Part model, mm, in its own coordinate system. A direction names the side the tool comes from. Give positions to 0.01 mm unless a question says otherwise; leave off trailing zeros. Write each loop counter-clockwise with the first axis right and the second up, starting at its lowest first coordinate (ties: lowest second). Pieces come first, ordered by that corner, then holes. Notation, with made-up numbers: M 64,28 L 69,28 A28 cw 69,63 Z; hole C -31,79 d2. An arc over 180 degrees is marked long. Use CSV: the item, a comma, the result in double quotes. Start each with the question number.
Item 1: Drill centre lines: line 1 (Z direction, x = -24, y = -1.5); line 2 (X direction, y = 1.5, z = -5); line 3 (X direction, y = 2.5, z = 6). Where is each one in solid material? Low to high. Write a range as [from, to].
Item 2: Which spindle directions (+Z, -Z, +X, -X, +Y, -Y) get a long thin tool onto all of the face, cutting with end or side? Do faces 1 (the cylindrical face through (10.165, -1.014, -9.699)), 2 (the flat face through (-10, 3, 9)), 3 (the cylindrical face through (-29.649, -1.014, -9.715)), 4 (the flat face through (-18, 10, 0)), 5 (the flat face through (-12, 9.5, 0)). Say none if no direction does.
Item 3: Mould opens along Z. For faces 6 (the cylindrical face through (13.5, 0.99, 4.93)), 7 (the cylindrical face through (10.165, 4.014, -9.699)), 8 (the flat face through (10.45, 4, 0)), 9 (the cylindrical face through (-37.215, 1.014, 9.699)) say: released by +Z, released by -Z, zero draft, split by the parting line, or undercut.
Item 4: Cut at B-B (y = -1). List the corners of the cut face in (x, z).
Item 5: Cut at A-A (x = -35). List the corners of the cut face in (y, z), then the cut area to 3 significant figures.
Item 6: Pin check, flat tips, straight feed: pin 1 (0.6 mm diameter, centred on x = -37.5, y = 1.5, fed in from -Z); pin 2 (1.7 mm diameter, centred on y = 3, z = 3.5, fed in from -X); pin 3 (4 mm diameter, centred on y = 6, z = -5.5, fed in from -X); pin 4 (3 mm diameter, centred on x = -35, z = -5, fed in from +Y). Stop position of each tip, or through.
from build123d import *

# Parameters (mm, degrees)
ESQUISSE1_W              = 38.4
ESQUISSE1_H              = 18
BOSS_EXTRU_1_DEPTH       = 2
ESQUISSE2_W              = 40.4
ESQUISSE2_H              = 20
ESQUISSE2_W_2            = 38.4
ESQUISSE2_H_2            = 18
BOSS_EXTRU_2_DEPTH       = 2
EXTRU_MINCE1_DEPTH       = 10
EXTRU_MINCE1_DEPTH_BACK  = 10
BOSS_EXTRU_3_DEPTH       = 1
ESQUISSE6_R              = 2.65
ENL_V_MAT_EXTRU_1_DEPTH  = 41.929818
BOSS_EXTRU_7_START       = -9
BOSS_EXTRU_7_DEPTH       = 18
BOSS_EXTRU_7_2_OUTLINE_W = 18
BOSS_EXTRU_7_2_OUTLINE_H = 0.5
BOSS_EXTRU_7_2_DEPTH     = 6.350393
BOSS_EXTRU_7_START_2     = 2.65
BOSS_EXTRU_7_3_OUTLINE_W = 18
BOSS_EXTRU_7_3_OUTLINE_H = 0.5
BOSS_EXTRU_7_3_DEPTH     = 6.35
BOSS_EXTRU_7_START_3     = 9.5
BOSS_EXTRU_7_4_DEPTH     = 0.5
BOSS_EXTRU_7_5_DEPTH     = 0.5
CONG_1_R                 = 1
ENL_V_MAT_EXTRU_2_DEPTH  = 44.453999


with BuildPart() as part:
    # Esquisse1 → Boss.-Extru.1 (new body)
    with BuildSketch(Plane(origin=(0, 0, 0), x_dir=(1, 0, 0), z_dir=(0, 1, 0))):
        with BuildLine():
            Line((-37.5, 10), (18, 10))
            Line((18, 10), (18, 6))
            Line((18, 6), (17.232051, 6))
            ThreePointArc((17.232051, 6), (13.5, 5), (17.232051, 4))
            Line((17.232051, 4), (18, 4))
            Line((18, 4), (18, -4))
            Line((18, -4), (17.232051, -4))
            ThreePointArc((17.232051, -4), (13.5, -5), (17.232051, -6))
            Line((17.232051, -6), (18, -6))
            Line((18, -6), (18, -10))
            Line((18, -10), (-37.5, -10))
            Line((-37.5, -10), (-37.5, -6))
            Line((-37.5, -6), (-36.732051, -6))
            ThreePointArc((-36.732051, -6), (-33, -5), (-36.732051, -4))
            Line((-36.732051, -4), (-37.5, -4))
            Line((-37.5, -4), (-37.5, 4))
            Line((-37.5, 4), (-36.732051, 4))
            ThreePointArc((-36.732051, 4), (-33, 5), (-36.732051, 6))
            Line((-36.732051, 6), (-37.5, 6))
            Line((-37.5, 6), (-37.5, 10))
        make_face()
        with Locations((-9.75, 0)):
            Rectangle(ESQUISSE1_W, ESQUISSE1_H, mode=Mode.SUBTRACT)
    extrude(amount=BOSS_EXTRU_1_DEPTH)

    # Esquisse2 → Boss.-Extru.2 (add)
    with BuildSketch(Plane.XZ):
        with Locations((-9.75, 0)):
            Rectangle(ESQUISSE2_W, ESQUISSE2_H)
        with Locations((-9.75, 0)):
            Rectangle(ESQUISSE2_W_2, ESQUISSE2_H_2, mode=Mode.SUBTRACT)
    extrude(amount=BOSS_EXTRU_2_DEPTH)

    # Esquisse3 → Extru.-Mince1 (add, two sides: drawn at the far end of the back side and taken through both)
    with BuildSketch(Plane.XY.offset(-EXTRU_MINCE1_DEPTH_BACK)):
        Polygon((-29.95, 2), (-29.95, 4.786585), (-17, 9.5), (7.45, 9.5), (10.45, 6.5), (10.45, 2), (9.45, 2), (9.45, 6.085786), (7.035786, 8.5), (-16.823673, 8.5), (-28.95, 4.086378), (-28.95, 2), align=None)
    extrude(amount=EXTRU_MINCE1_DEPTH + EXTRU_MINCE1_DEPTH_BACK)

    # Esquisse4 → Boss.-Extru.3 (add)
    with BuildSketch(Plane.XY.offset(10)):
        Polygon((10.45, 6.5), (10.45, 2), (-29.95, 2), (-29.95, 4.786585), (-17, 9.5), (7.45, 9.5), align=None)
    boss_extru_3 = extrude(amount=-BOSS_EXTRU_3_DEPTH)

    # Symétrie1: Boss.-Extru.3 across plane
    add(boss_extru_3.mirror(Plane.XY))

    # Esquisse5 → Révolution1 (revolve)
    with BuildSketch(Plane.XY, mode=Mode.PRIVATE) as r_volution1_sk:
        Polygon((-6.25, 9.5), (-4.75, 11), (0, 11), (0, 10), (-4.335786, 10), (-5.542893, 8.792893), align=None)
    revolve(r_volution1_sk.sketch.rotate(Axis((0, 11, 0), (0, -1, 0)), 270), axis=Axis((0, 11, 0), (0, -1, 0)))

    # Esquisse6 → Enlèv. mat.-Extru.1 (cut, through all)
    with BuildSketch(Plane(origin=(0, 11, 0), x_dir=(1, 0, 0), z_dir=(0, 1, 0))):
        Circle(ESQUISSE6_R)
    extrude(amount=-ENL_V_MAT_EXTRU_1_DEPTH, mode=Mode.SUBTRACT)

    # Boss.-Extru.7: read off the stored shape, not the designer's step
    # Boss.-Extru.7 outline → Boss.-Extru.7 (add)
    with BuildSketch(Plane.XY.offset(BOSS_EXTRU_7_START)):
        Polygon((-12.5, 10), (-26.95, 10), (-26.95, 5.878496), (-17, 9.5), (-12.5, 9.5), align=None)
    extrude(amount=BOSS_EXTRU_7_DEPTH)

    # Boss.-Extru.7 2 outline → Boss.-Extru.7 2 (add)
    with BuildSketch(Plane.XY.offset(BOSS_EXTRU_7_START)):
        with Locations((-2.5, 9.75)):
            Rectangle(BOSS_EXTRU_7_2_OUTLINE_W, BOSS_EXTRU_7_2_OUTLINE_H)
    extrude(amount=BOSS_EXTRU_7_2_DEPTH)

    # Boss.-Extru.7 3 outline → Boss.-Extru.7 3 (add)
    with BuildSketch(Plane.XY.offset(BOSS_EXTRU_7_START_2)):
        with Locations((-2.5, 9.75)):
            Rectangle(BOSS_EXTRU_7_3_OUTLINE_W, BOSS_EXTRU_7_3_OUTLINE_H)
    extrude(amount=BOSS_EXTRU_7_3_DEPTH)

    # Boss.-Extru.7 4 outline → Boss.-Extru.7 4 (cut)
    with BuildSketch(Plane(origin=(0, 0, 0), x_dir=(1, 0, 0), z_dir=(0, 1, 0)).offset(BOSS_EXTRU_7_START_3)):
        with BuildLine():
            Line((-0.04562, 2.649607), (0.04562, 2.649607))
            ThreePointArc((0.04562, 2.649607), (0, 2.65), (-0.04562, 2.649607))
        make_face()
    extrude(amount=BOSS_EXTRU_7_4_DEPTH, mode=Mode.SUBTRACT)

    # Boss.-Extru.7 5 outline → Boss.-Extru.7 5 (add)
    with BuildSketch(Plane(origin=(0, 0, 0), x_dir=(1, 0, 0), z_dir=(0, 1, 0)).offset(BOSS_EXTRU_7_START_3)):
        with BuildLine():
            ThreePointArc((0.04562, 2.649607), (2.649902, -0.022811), (0, -2.65))
            Line((0, -2.65), (6.5, -2.65))
            Line((6.5, -2.65), (6.5, 2.649607))
            Line((6.5, 2.649607), (0.04562, 2.649607))
        make_face()
        with BuildLine():
            Line((-11.5, -2.65), (0, -2.65))
            ThreePointArc((0, -2.65), (-2.649902, -0.022811), (-0.04562, 2.649607))
            Line((-0.04562, 2.649607), (-11.5, 2.649607))
            Line((-11.5, 2.649607), (-11.5, -2.65))
        make_face()
    extrude(amount=BOSS_EXTRU_7_5_DEPTH)

    # Congé1
    cong_1_edges = [part.edges().sort_by_distance(p)[0] for p in [
        (-29.95, 4.786585, 0),
        (-23.475, 7.143293, -10),
        (-23.475, 7.143293, 10),
        (-4.775, 9.5, 10),
        (-4.775, 9.5, -10),
        (7.45, 9.5, 0),
        (10.45, 6.5, 0),
        (8.95, 8, 10),
        (8.95, 8, -10),
        (10.45, 4.25, 10),
        (10.45, 4.25, -10),
        (18, 1, -10),
        (18, 1, 10),
        (10.45, -1, 10),
        (-29.95, -1, 10),
        (-29.95, 3.393293, 10),
        (-29.95, 3.393293, -10),
        (-29.95, -1, -10),
        (-37.5, 1, -10),
        (-37.5, 1, 10),
        (10.45, -1, -10),
    ]]
    fillet(cong_1_edges, radius=CONG_1_R - 0.0001)  # a hair under: the kernel refuses the full size

    # Esquisse11 → Enlèv. mat.-Extru.2 (cut, through all)
    with BuildSketch(Plane(origin=(0, 0, -9), x_dir=(-1, 0, 0), z_dir=(0, 0, -1))):
        Polygon((26.95, 5.878496), (21.455546, 11.37295), (30.404027, 11.37295), align=None)
    extrude(amount=-ENL_V_MAT_EXTRU_2_DEPTH, mode=Mode.SUBTRACT)


solid = part.part
Worked answers:
1,line 1,"z = [-10, -9], [9, 10]"
1,line 2,"x = [-33, -28.95], [9.45, 13.5]"
1,line 3,"x = [-29.95, -28.95], [9.45, 10.45]"
2,face 1,"-Z, +X, -Y"
2,face 2,"-Y"
2,face 3,"-Z, -X, -Y"
2,face 4,"+Z, -Z, -X, +Y"
2,face 5,"+Z, -Z, +Y"
3,face 6,"undercut"
3,face 7,"released by -Z"
3,face 8,"zero draft"
3,face 9,"released by +Z"
4,outline,"M -29.95,-9 A1 ccw -28.95,-10 L 9.45,-10 A1 ccw 10.45,-9 L 10.45,9 A1 ccw 9.45,10 L -28.95,10 A1 ccw -29.95,9 Z; hole M -28.95,-9 L 9.45,-9 L 9.45,9 L -28.95,9 Z"
5,outline,"M 0,-10 L 2,-10 L 2,-7 L 0,-7 Z; M 0,-3 L 2,-3 L 2,3 L 0,3 Z; M 0,7 L 2,7 L 2,10 L 0,10 Z"
5,area,"24.0 mm^2"
6,pin 1,"stops at z = -9.71"
6,pin 2,"stops at x = -29.95"
6,pin 3,"stops at x = -29.95"
6,pin 4,"passes through"
